Geometry check sheet. Reference: the model listing, model coordinates, mm. A direction names the side the tool comes from. Round coordinates to 2 decimals unless told otherwise and drop trailing zeros. Write each loop counter-clockwise with the first axis right and the second up, starting at its lowest first coordinate (ties: lowest second). Pieces come first, ordered by that corner, then holes.
from build123d import *

# Parameters (mm, degrees)
BOSS_EXTRUDE1_DEPTH = 20
BOSS_EXTRUDE2_DEPTH = 15
CUT_EXTRUDE1_DEPTH  = 5
SKETCH5_R           = 2.5
CUT_EXTRUDE2_DEPTH  = 3


with BuildPart() as part:
    # Sketch1 → Boss-Extrude1 (new body)
    with BuildSketch(Plane.XY):
        with BuildLine():
            Line((-25, 10), (25, 10))
            Line((25, 10), (25, -10))
            Line((25, -10), (22, -15))
            ThreePointArc((22, -15), (21, -15.414213562), (20, -15))
            ThreePointArc((20, -15), (0, -5.003320801), (-20, -15))
            ThreePointArc((-20, -15), (-21.018204397, -15.363175427), (-21.994987437, -14.9))
            Line((-21.994987437, -14.9), (-25, -10))
            Line((-25, -10), (-25, 10))
        make_face()
    extrude(amount=BOSS_EXTRUDE1_DEPTH)

    # Sketch2 → Boss-Extrude2 (add)
    with BuildSketch(Plane.XY.offset(20)):
        Polygon((0, 10), (-8, 10), (-8, 2), (8, 2), (8, 10), align=None)
    extrude(amount=BOSS_EXTRUDE2_DEPTH)

    # Sketch4 → Cut-Extrude1 (cut)
    with BuildSketch(Plane.XZ.offset(-2)):
        Polygon((2.457286371, 23.755949434), (4.900734659, 28.011873987), (2.436720023, 32.255924553), (-2.4707429, 32.244050566), (-4.914191188, 27.988126013), (-2.450176552, 23.744075447), align=None)
    extrude(amount=-CUT_EXTRUDE1_DEPTH, mode=Mode.SUBTRACT)

    # Sketch5 → Cut-Extrude2 (cut)
    with BuildSketch(Plane.XZ.offset(-7)):
        with Locations((0, 28.00001244)):
            Circle(SKETCH5_R)
    extrude(amount=-CUT_EXTRUDE2_DEPTH, mode=Mode.SUBTRACT)


solid = part.part
1. Scan lines: line 1 along Z through (x, y) = (0, 8.4); line 2 along Z through (x, y) = (-18.5, -7.5); line 3 along X through (y, z) = (6.25, 32.5). Record each from-to range of solid material in increasing order.
2. Access from +Z, -Z, +X, -X, +Y, -Y to the whole of each face (thin tool, end or side, straight path). Record for faces 1 (the face through (-3.7, 4.5, 25.9)), 2 (the face through (8, 6, 27)), 3 (the face through (-4, 2, 26)).
3. Section check B-B (x = 0). Record the cut outline in (y, z), plus the area to 3 significant figures.
4. Release check for a two-part mould opening along Z. For faces 4 (the face through (2, 7, 26)), 5 (the face through (-23.48, -12.48, 9.86)), 6 (the face through (0, 6, 35)) record: +Z half, -Z half, draft (parallel to the pull), parting line (faces both ways), or undercut.
5. Section check C-C (z = 8). Record the cut outline in (x, y), plus the area to 3 significant figures.
6. Section check D-D (y = 8.25). Record the cut outline in (x, z).
7. Section check A-A (y = -13). Record the cut outline in (x, z).
8. Depth check by flat-ended pin: pin 1 Ø6 at (x, z) = (1, 9.5) entering from -Y; pin 2 Ø2.5 at (y, z) = (6.5, 27) entering from +X; pin 3 Ø8 at (x, z) = (-18.5, 11.5) entering from -Y. Enter the tip coordinate at first touch or a pass-through.
Results below:
1. line 1: z = 0 to 25.5, 30.5 to 35
1. line 2: z = 0 to 20
1. line 3: x = -8 to 8
2. face 1: -Y
2. face 2: +Z, +X, +Y, -Y
2. face 3: +Z, +X, -X, -Y
3. outline: (-5, 0) - (10, 0) - (10, 25.5) - (7, 25.5) - (7, 23.75) - (2, 23.75) - (2, 20) - (-5, 20) - close; (2, 32.25) - (7, 32.25) - (7, 30.5) - (10, 30.5) - (10, 35) - (2, 35) - close
3. area: 363 mm2
4. face 4: undercut
4. face 5: draft
4. face 6: +Z half
5. outline: (-25, -10) - (-21.99, -14.9) arc R1.41 ccw to (-20, -15) arc R25 cw to (20, -15) arc R1.41 ccw to (22, -15) - (25, -10) - (25, 10) - (-25, 10) - close
5. area: 956 mm2
6. outline: (-25, 0) - (25, 0) - (25, 20) - (8, 20) - (8, 35) - (-8, 35) - (-8, 20) - (-25, 20) - close; hole circle Ø5 at (0, 28)
7. outline: (-23.16, 0) - (-18.33, 0) - (-18.33, 20) - (-23.16, 20) - close; (18.33, 0) - (23.2, 0) - (23.2, 20) - (18.33, 20) - close
8. pin 1: stops at y = -5.33
8. pin 2: stops at x = 8
8. pin 3: stops at y = -15.36
